from build123d import *

# Parameters (mm, degrees)
CUT_EXTRUDE1_DEPTH      = 135.59847696
CUT_EXTRUDE1_DEPTH_BACK = 135.59847696
SKETCH3_R               = 4
FILLET1_R               = 2.5


with BuildPart() as part:
    # Sketch1 → Revolve1 (revolve)
    with BuildSketch(Plane(origin=(0, 0, 0), x_dir=(1, 0, 0), z_dir=(0, 1, 0))):
        Polygon((-127.5, 0), (127.5, 0), (127.5, -6), (123.5, -6), (123.5, -10), (118.5, -17), (118.5, -25.3), (113.5, -25.3), (113.5, -25.4), (-86.5, -25.4), (-86.5, -25.3), (-91.5, -25.3), (-91.5, -20), (-106.2, -20), (-106.2, -30.5), (-113, -30.5), (-113, -18.75), (-118.5, -18.75), (-118.5, -17), (-123.5, -10), (-123.5, -6), (-127.5, -6), align=None)
    revolve(axis=Axis((-127.5, 0, 0), (1, 0, 0)))

    # Sketch3 → Cut-Extrude1 (cut, two sides: drawn at the far end of the back side and taken through both)
    with BuildSketch(Plane(origin=(0, 0, 0), x_dir=(0, 0, -1), z_dir=(1, 0, 0)).offset(-CUT_EXTRUDE1_DEPTH_BACK)):
        Circle(SKETCH3_R)
    extrude(amount=CUT_EXTRUDE1_DEPTH + CUT_EXTRUDE1_DEPTH_BACK, mode=Mode.SUBTRACT)

    # Fillet1
    fillet1_edges = [part.edges().sort_by_distance(p)[0] for p in [
        (-91.5, 0, -25.3),
        (118.5, 0, -25.3),
    ]]
    fillet(fillet1_edges, radius=FILLET1_R)


solid = part.part
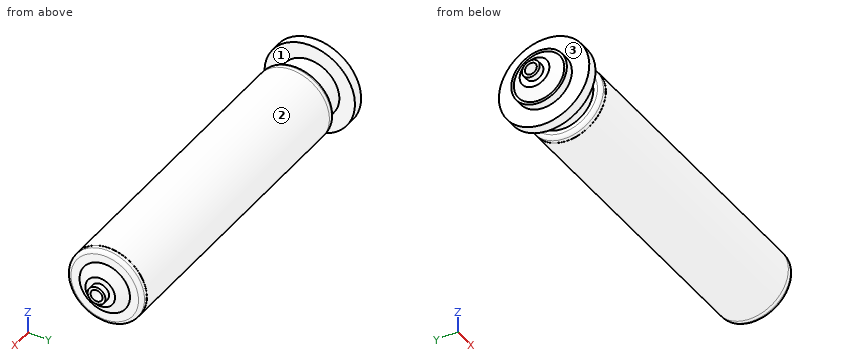
Build history of the part. All positions in model axes, mm. Face numbers are marked on the shaded views. Round coordinates to 2 decimals unless told otherwise and drop trailing zeros. Write each loop counter-clockwise with the first axis right and the second up, starting at its lowest first coordinate (ties: lowest second). Pieces come first, ordered by that corner, then holes. Notation, with made-up numbers: M 35.25,66 L 41.25,66 A22 cw 41.25,93 Z; hole C 7,42 d4. An arc over 180 degrees is marked long. Answer in a Markdown table with one row per item.
1. Mould opens along X. For the marked faces 1, 2 and 3 say: +X half, -X half, draft (parallel to the pull), parting line (faces both ways), or undercut.
Geometry check:
| item | result |
|---|---|
| face 1 | undercut |
| face 2 | draft |
| face 3 | -X half |
2. Saw through at A-A (x = 23.5). List the corners of the cut face in (y, z).
Geometry check:
| item | result |
|---|---|
| outline | C 0,0 d50.8; hole C 0,0 d8 |
3. Probe L1, parallel to Y at x = 24.5, z = 0.5; L2, parallel to Z at x = 6.5, y = 0; L3, parallel to X at y = 21, z = 0. List the from-to ranges inside material, lowest first. Write a range as [from, to].
Geometry check:
| item | result |
|---|---|
| L1 | [-25.4, -3.97], [3.97, 25.4] |
| L2 | [-25.4, -4], [4, 25.4] |
| L3 | [-113, -106.2], [-91.5, 118.5] |
4. Flat gauge pins, fed straight in: P1, Ø12, axis at x = -41.5, y = 15, coming from the +Z side; P2, Ø2, axis at x = -88, y = -11.5, coming from the +Z side; P3, Ø5, axis at y = 0, z = 0, coming from the +X side; P4, Ø4, axis at y = 22, z = 17, coming from the -X side. Where does each tip first touch, or does it go through?
Geometry check:
| item | result |
|---|---|
| P1 | z = 23.75 |
| P2 | z = 23.02 |
| P3 | through |
| P4 | x = -113 |
